```python
from build123d import *

# Parameters (mm, degrees)
STOCK_GOUX_START         = 56.852102372
STOCK_GOUX_LIKED_1_DEPTH = 33.663747278
BOSS_EXTRUDE1_DEPTH      = 33.663747
BOSS_EXTRUDE2_DEPTH      = 4
BOSS_EXTRUDE3_DEPTH      = 4
SKETCH4_R                = 0.64999997
CUT_EXTRUDE1_DEPTH       = 152.446320344
CUT_EXTRUDE2_DEPTH       = 0.4
SKETCH6_R                = 1.5
CUT_EXTRUDE3_DEPTH       = 5.08


# Read off the part's stored shape, not the designer's step: Stock-Goux Liked-1
with BuildPart() as part:
    # Stock-Goux Liked-1 outline → Stock-Goux Liked-1 (new body)
    with BuildSketch(Plane.YZ.offset(STOCK_GOUX_START)):
        Polygon((-51.598102466, 113.704878), (-51.598102466, 110.204877888), (-56.598102372, 110.204877888), (-56.598102372, 109.704877872), (-45.441248273, 109.704877872), (-37.552161083, 117.593965062), (-37.905714485, 117.947518464), (-41.441248325, 114.411984624), (-43.916122138, 116.886858438), (-47.098102576, 113.704878), align=None)
    extrude(amount=STOCK_GOUX_LIKED_1_DEPTH)

    # Sketch1 → Boss-Extrude1 (add)
    with BuildSketch(Plane(origin=(90.51584965, 0, 0), x_dir=(0, 0, -1), z_dir=(1, 0, 0))):
        Polygon((-109.704877872, -45.441248273), (-109.704877872, -37.552161083), (-117.593965062, -37.552161083), align=None)
    extrude(amount=-BOSS_EXTRUDE1_DEPTH)

    # Sketch2 → Boss-Extrude2 (add)
    with BuildSketch(Plane.ZY.offset(-56.852102372)):
        Polygon((113.704878, -47.098102576), (109.704877872, -47.098102576), (109.704877872, -37.552161083), (117.593965062, -37.552161083), (117.947518464, -37.905714485), (114.411984624, -41.441248325), (116.886858438, -43.916122138), align=None)
    extrude(amount=BOSS_EXTRUDE2_DEPTH)

    # Sketch3 → Boss-Extrude3 (add)
    with BuildSketch(Plane(origin=(90.51584965, 0, 0), x_dir=(0, 0, -1), z_dir=(1, 0, 0))):
        Polygon((-113.704878, -47.098102576), (-109.704877872, -47.098102576), (-109.704877872, -37.552161083), (-117.593965062, -37.552161083), (-117.947518464, -37.905714485), (-114.411984624, -41.441248325), (-116.886858438, -43.916122138), align=None)
    extrude(amount=BOSS_EXTRUDE3_DEPTH)

    # Sketch4 → Cut-Extrude1 (cut, through all)
    with BuildSketch(Plane.XZ.offset(47.098102576)):
        with Locations(Location((92.51584965, 111.954877944, 0), (0, 0, 270))):
            Circle(SKETCH4_R)
    cut_extrude1 = extrude(amount=-CUT_EXTRUDE1_DEPTH, mode=Mode.SUBTRACT)

    # Mirror2: Cut-Extrude1 across plane
    add(cut_extrude1.mirror(Plane(origin=(73.683976011, 0, 0), x_dir=(0, 0, 1), z_dir=(1, 0, 0))), mode=Mode.SUBTRACT)

    # Sketch5 → Cut-Extrude2 (cut)
    with BuildSketch(Plane(origin=(0, 0, 109.704877872), x_dir=(-1, 0, 0), z_dir=(0, 0, -1))):
        with BuildLine():
            Line((-76.075617186, -43.318922194), (-76.075617186, -43.888793989))
            add(Edge.make_bspline(
                [(-76.075617186, -43.888793989), (-76.139538978, -43.873355233), (-76.264500854, -43.843173727), (-76.443039741, -43.780222416), (-76.611992416, -43.711643767), (-76.768195292, -43.629294963), (-76.914787587, -43.539471937), (-77.048444427, -43.436560714), (-77.172565093, -43.325309217), (-77.282716253, -43.202255381), (-77.382461562, -43.073207666), (-77.467506308, -42.936347713), (-77.540665843, -42.794429035), (-77.600936835, -42.646468351), (-77.646340285, -42.492025153), (-77.679281918, -42.332495694), (-77.700674368, -42.167461915), (-77.702762181, -42.055434144), (-77.703822314, -41.998549598)],
                knots=[0, 0, 0, 0, 1.162005537, 2.271625781, 3.343758855, 4.383309926, 5.390229558, 6.379919256, 7.361854164, 8.333198761, 9.295911338, 10.242430842, 11.177959212, 12.116337295, 13.062827104, 14.020064771, 14.994644689, 16, 16, 16, 16], degree=3))
            add(Edge.make_bspline(
                [(-77.703822314, -41.998549598), (-77.701319996, -41.915668052), (-77.696369943, -41.751712846), (-77.651168037, -41.510842747), (-77.579639583, -41.278565518), (-77.480808678, -41.057423597), (-77.358911695, -40.852013012), (-77.213832816, -40.669248788), (-77.048371226, -40.511608204), (-76.865613573, -40.379356976), (-76.670295721, -40.27580662), (-76.469272578, -40.199449914), (-76.263021002, -40.152964864), (-76.123761367, -40.146940425), (-76.053992586, -40.143922194)],
                knots=[0, 0, 0, 0, 1.083050992, 2.142477498, 3.193116406, 4.255571735, 5.30263384, 6.308962982, 7.297363603, 8.282367274, 9.249857812, 10.179914175, 11.08814088, 12, 12, 12, 12], degree=3))
            add(Edge.make_bspline(
                [(-76.053992586, -40.143922194), (-75.986851687, -40.146033281), (-75.855467367, -40.15016435), (-75.663658365, -40.185241216), (-75.482880033, -40.244271293), (-75.312371353, -40.326040719), (-75.15321343, -40.43188896), (-75.00504817, -40.560109425), (-74.867218412, -40.711607111), (-74.788261654, -40.826413184), (-74.747612378, -40.885518749)],
                knots=[0, 0, 0, 0, 1.024540389, 2.004866551, 2.965041327, 3.920577974, 4.882998113, 5.874504559, 6.905732034, 8, 8, 8, 8], degree=3))
            add(Edge.make_bspline(
                [(-74.747612378, -40.885518749), (-74.715113083, -40.817883608), (-74.650618225, -40.683661659), (-74.522124234, -40.502557078), (-74.377408106, -40.335645539), (-74.263212693, -40.243656204), (-74.205725359, -40.197347675)],
                knots=[0, 0, 0, 0, 1.015663554, 2.015584519, 3.001021554, 4, 4, 4, 4], degree=3))
            add(Edge.make_bspline(
                [(-74.205725359, -40.197347675), (-74.163892009, -40.166792668), (-74.080910361, -40.106183014), (-73.947494274, -40.031369974), (-73.812599429, -39.963499153), (-73.672610221, -39.910612326), (-73.529149182, -39.869656882), (-73.381969977, -39.840381509), (-73.230952422, -39.822194854), (-73.128785494, -39.819590352), (-73.077430086, -39.818281169)],
                knots=[0, 0, 0, 0, 1.025084078, 2.033381695, 3.024893161, 4.013698104, 4.991890475, 5.976764909, 6.982997093, 8, 8, 8, 8], degree=3))
            add(Edge.make_bspline(
                [(-73.077430086, -39.818281169), (-72.988512904, -39.821537398), (-72.811096985, -39.828034533), (-72.548971743, -39.88609203), (-72.292774916, -39.976132066), (-72.04760793, -40.103855132), (-71.81844159, -40.260217785), (-71.611884948, -40.444185319), (-71.437120387, -40.658387778), (-71.289330919, -40.895062092), (-71.172293376, -41.152579903), (-71.08793697, -41.426890731), (-71.037340068, -41.716407105), (-71.031268974, -41.914392881), (-71.028181288, -42.015086057)],
                knots=[0, 0, 0, 0, 0.955697303, 1.906897079, 2.875188111, 3.870982192, 4.871999088, 5.854111427, 6.836107184, 7.836239895, 8.848948182, 9.870701427, 10.917064451, 12, 12, 12, 12], degree=3))
            add(Edge.make_bspline(
                [(-71.028181288, -42.015086057), (-71.029770214, -42.082971085), (-71.03289669, -42.216546184), (-71.053889344, -42.412991677), (-71.093273096, -42.600110727), (-71.142803615, -42.779720334), (-71.211285106, -42.949109752), (-71.292927731, -43.110715491), (-71.389825107, -43.263829176), (-71.502140187, -43.407541515), (-71.627860123, -43.541698969), (-71.769073476, -43.662883652), (-71.923144715, -43.772436343), (-72.091459735, -43.869660957), (-72.273547112, -43.954966676), (-72.4701365, -44.026517714), (-72.679703854, -44.088990608), (-72.825706955, -44.118093073), (-72.900617186, -44.133024759)],
                knots=[0, 0, 0, 0, 1.048603596, 2.063302207, 3.045874044, 3.999447474, 4.937100059, 5.862643889, 6.7929026, 7.7308982, 8.676022965, 9.627908155, 10.600123445, 11.591992905, 12.626222643, 13.701663232, 14.820785756, 16, 16, 16, 16], degree=3))
            Line((-72.900617186, -44.133024759), (-72.900617186, -43.563152964))
            add(Edge.make_bspline(
                [(-72.900617186, -43.563152964), (-72.851723976, -43.548306135), (-72.756622436, -43.519427763), (-72.619752167, -43.470270966), (-72.494279699, -43.414267101), (-72.379284606, -43.35418783), (-72.27363439, -43.291089792), (-72.180122714, -43.220486999), (-72.094642275, -43.147608693), (-72.046482765, -43.092673295), (-72.022912859, -43.065787178)],
                knots=[0, 0, 0, 0, 1.198163088, 2.33053128, 3.407730985, 4.417276592, 5.372219308, 6.28897303, 7.162600585, 8, 8, 8, 8], degree=3))
            add(Edge.make_bspline(
                [(-72.022912859, -43.065787178), (-71.995513327, -43.030229419), (-71.94079884, -42.959223657), (-71.870776253, -42.843589465), (-71.810838593, -42.721552229), (-71.762118751, -42.592094244), (-71.72554788, -42.455198144), (-71.699225888, -42.311419238), (-71.681849284, -42.16052162), (-71.680270254, -42.057536944), (-71.679463339, -42.004909775)],
                knots=[0, 0, 0, 0, 0.946083416, 1.889246487, 2.84504177, 3.809995578, 4.801312957, 5.829064617, 6.89060985, 8, 8, 8, 8], degree=3))
            add(Edge.make_bspline(
                [(-71.679463339, -42.004909775), (-71.680580768, -41.945485563), (-71.682765802, -41.829286646), (-71.702860298, -41.65973283), (-71.732125477, -41.498429318), (-71.777324746, -41.34716701), (-71.833170005, -41.203964518), (-71.903289255, -41.070829239), (-71.985557536, -40.946013447), (-72.079064295, -40.831115811), (-72.181429007, -40.72780039), (-72.288495579, -40.636832988), (-72.399812584, -40.559499673), (-72.515996032, -40.497118038), (-72.636564804, -40.447859183), (-72.761857252, -40.414325376), (-72.890848006, -40.391009056), (-72.978530564, -40.389110202), (-73.02273257, -40.388152964)],
                knots=[0, 0, 0, 0, 1.217147791, 2.380027433, 3.494444702, 4.572153297, 5.609568379, 6.639424714, 7.649109417, 8.668170816, 9.669597737, 10.625200337, 11.543417969, 12.441394052, 13.322311151, 14.205496177, 15.095365482, 16, 16, 16, 16], degree=3))
            add(Edge.make_bspline(
                [(-73.02273257, -40.388152964), (-73.081895072, -40.39093521), (-73.199925692, -40.396485859), (-73.3736414, -40.438686775), (-73.541075629, -40.508726152), (-73.700059811, -40.604856525), (-73.845611274, -40.724738389), (-73.976406445, -40.862703865), (-74.084229706, -41.022506322), (-74.158794458, -41.169475897), (-74.209659091, -41.299681811), (-74.243541433, -41.411106059), (-74.272231733, -41.535850429), (-74.298924055, -41.672405015), (-74.321641341, -41.821799159), (-74.340585783, -41.98387009), (-74.355744213, -42.158650688), (-74.362513486, -42.279647517), (-74.366001801, -42.341999118)],
                knots=[0, 0, 0, 0, 1.070505987, 2.135685285, 3.216438728, 4.346150463, 5.486482244, 6.621737109, 7.7759408, 8.963942283, 9.59839197, 10.305095457, 11.070459627, 11.915156775, 12.823989992, 13.805807174, 14.869297358, 16, 16, 16, 16], degree=3))
            Line((-74.366001801, -42.341999118), (-75.017283852, -42.341999118))
            add(Edge.make_bspline(
                [(-75.017283852, -42.341999118), (-75.018809153, -42.263466821), (-75.021795797, -42.109695136), (-75.050669999, -41.884479267), (-75.097024447, -41.670033169), (-75.16325695, -41.469439558), (-75.24127084, -41.286958717), (-75.331413736, -41.128005999), (-75.433440936, -40.996765899), (-75.545399019, -40.891867311), (-75.664822791, -40.812137014), (-75.790055878, -40.75479729), (-75.921594744, -40.720622764), (-76.011397636, -40.716078263), (-76.056536657, -40.713793989)],
                knots=[0, 0, 0, 0, 1.322091412, 2.58874672, 3.817242262, 5.011895168, 6.140903042, 7.155122731, 8.080855046, 8.929742606, 9.727943956, 10.488587771, 11.240295418, 12, 12, 12, 12], degree=3))
            add(Edge.make_bspline(
                [(-76.056536657, -40.713793989), (-76.089703227, -40.714529395), (-76.155686544, -40.715992449), (-76.252389139, -40.735176783), (-76.346131292, -40.762679558), (-76.435844182, -40.802610281), (-76.521711422, -40.85434671), (-76.604674968, -40.916751009), (-76.683662816, -40.991601722), (-76.75908247, -41.075435333), (-76.827693483, -41.168266491), (-76.887739473, -41.267929765), (-76.938677009, -41.37402103), (-76.980820221, -41.485860698), (-77.012486847, -41.603969954), (-77.03523311, -41.727750359), (-77.049452113, -41.857450016), (-77.051499485, -41.945935793), (-77.052540263, -41.990917387)],
                knots=[0, 0, 0, 0, 0.884325644, 1.759323928, 2.622595547, 3.489424008, 4.37295195, 5.294616785, 6.255907374, 7.274251867, 8.302369084, 9.333474657, 10.37669385, 11.44084034, 12.520297356, 13.637342342, 14.798947025, 16, 16, 16, 16], degree=3))
            add(Edge.make_bspline(
                [(-77.052540263, -41.990917387), (-77.050015934, -42.063219699), (-77.045085334, -42.20444293), (-77.001899867, -42.408032851), (-76.932996773, -42.597297928), (-76.850749723, -42.741966652), (-76.76955965, -42.848796465), (-76.698653035, -42.925136053), (-76.619853483, -43.000103265), (-76.528307574, -43.068766136), (-76.430214969, -43.138206065), (-76.320589147, -43.201424055), (-76.202289746, -43.262855211), (-76.118659094, -43.299871265), (-76.075617186, -43.318922194)],
                knots=[0, 0, 0, 0, 1.472543308, 2.876219568, 4.221790263, 5.565193594, 6.249813518, 6.953379497, 7.687249741, 8.463570142, 9.283606569, 10.136032583, 11.040678096, 12, 12, 12, 12], degree=3))
        make_face()
    extrude(amount=-CUT_EXTRUDE2_DEPTH, mode=Mode.SUBTRACT)

    # Sketch6 → Cut-Extrude3 (cut)
    with BuildSketch(Plane(origin=(0, -37.552161083, 0), x_dir=(1, 0, 0), z_dir=(0, 1, 0))):
        with Locations(Location((54.852102372, -111.954877944, 0), (0, 0, 270))):
            Circle(SKETCH6_R)
        with Locations(Location((92.51584965, -111.954877944, 0), (0, 0, 270))):
            Circle(SKETCH6_R)
    extrude(amount=-CUT_EXTRUDE3_DEPTH, mode=Mode.SUBTRACT)


solid = part.part
```
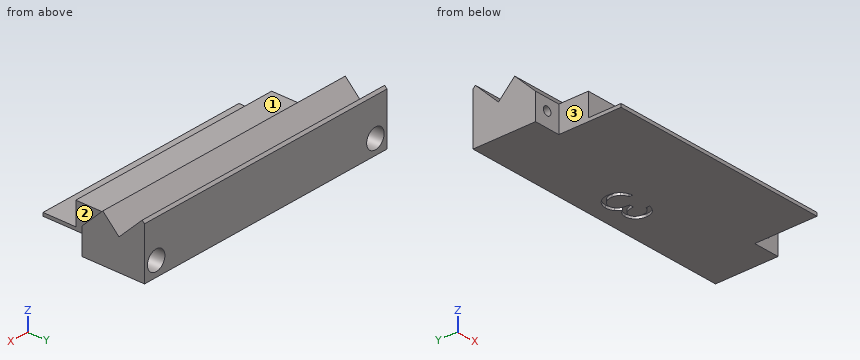
Check sheet for the modelled part. Datum: model origin and axes. Units: mm. Face numbers are marked on the shaded views. A direction names the side the tool comes from. Round coordinates to 2 decimals unless told otherwise and drop trailing zeros. Loops run counter-clockwise (first coordinate to the right, second up) from the corner with the lowest first, then second, coordinate; pieces in that order, holes last. Notation, with made-up numbers: (-37, 70) - (16, 70) arc R10 ccw to (16, 85) - close; hole circle Ø2 at (46.25, -28). An arc over 180 degrees is marked (long way). Answer as a JSON object with one key per item and string values. Group by question number.
Q1. Scan lines: line 1 along Z through (x, y) = (70.5, -51.5); line 2 along X through (y, z) = (-47.75, 111.25); line 3 along X through (y, z) = (-42, 112.75). Record each from-to range of solid material in increasing order. Write a range as [from, to].
Q2. Set-up check for the marked faces 1, 2 and 3: record each of +Z, -Z, +X, -X, +Y, -Y from which the full face is reachable in a straight line by a thin tool's end or side.
Q3. Sectioned sample at D-D, the plane y = -39. Enter the section's corners in (x, z).
Q4. Gauge pin test, flat ends, axial feed: P1, Ø1.5, axis at x = 64, z = 115, coming from the -Y side; P2, Ø1.2, axis at x = 54.85, z = 111.95, coming from the +Y side; P3, Ø2.5, axis at x = 92.5, z = 112, coming from the +Y side; P4, Ø4, axis at x = 66, z = 112.5, coming from the -Y side. Record the tip position at first contact, or that the pin passes through.
Q5. Sectioned sample at B-B, the plane y = -45.25. Enter the section's corners in (x, z), plus the area to 3 significant figures.
Q6. Sectioned sample at C-C, the plane y = -48.25. Enter the section's corners in (x, z), plus the area to 3 significant figures.
Q7. Sectioned sample at A-A, the plane x = 87.5. Enter the section's corners in (y, z).
Solution:
{
 "1": {"line 1": "z = [109.7, 113.7]", "line 2": "x = [56.85, 90.52]", "line 3": "x = [52.85, 53.58], [56.12, 91.24], [93.79, 94.52]"},
 "2": {"face 1": "+Z, +X, -X, -Y", "face 2": "+Z, -Z, +X, -Y", "face 3": "+Z, -Z, -X, -Y"},
 "3": {"outline": "(52.85, 109.7) - (94.52, 109.7) - (94.52, 116.85) - (52.85, 116.85) - close; hole circle Ø3 at (54.85, 111.95); hole circle Ø3 at (92.52, 111.95)"},
 "4": {"P1": "stops at y = -46.55", "P2": "passes through", "P3": "stops at y = -42.63", "P4": "stops at y = -51.6"},
 "5": {"outline": "(52.85, 109.7) - (94.52, 109.7) - (94.52, 115.55) - (52.85, 115.55) - close; hole circle Ø1.3 at (54.85, 111.95); hole circle Ø1.3 at (92.52, 111.95)", "area": "241 mm²"},
 "6": {"outline": "(56.85, 109.7) - (90.52, 109.7) - (90.52, 113.7) - (56.85, 113.7) - close", "area": "135 mm²"},
 "7": {"outline": "(-56.6, 109.7) - (-37.55, 109.7) - (-37.55, 117.59) - (-37.91, 117.95) - (-41.44, 114.41) - (-43.92, 116.89) - (-47.1, 113.7) - (-51.6, 113.7) - (-51.6, 110.2) - (-56.6, 110.2) - close"}
}
